from build123d import *

# Parameters (mm, degrees)
F2_R = 15
F3_R = 2


with BuildPart() as f1:
    # F0 (on Front) → F1 (revolve)
    with BuildSketch(Plane.XZ):
        Polygon((-36, -25), (-32.5, -25), (-32.5, -5), (-25.5, 5), (-25.5, 25), (-29, 25), (-29, 5), (-36, -5), align=None)
    revolve(axis=Axis((0, 0, 12.5), (0, 0, 1)))

    # F2
    f2_edges = [f1.edges().sort_by_distance(p)[0] for p in [
        (29, 0, 5),
        (36, 0, -5),
        (25.5, 0, 5),
        (32.5, 0, -5),
    ]]
    fillet(f2_edges, radius=F2_R)

    # F3
    f3_edges = [f1.edges().sort_by_distance(p)[0] for p in [
        (29, 0, 25),
    ]]
    fillet(f3_edges, radius=F3_R)


solid = f1.part
Part model, mm, in its own coordinate system. A direction names the side the tool comes from. Give positions to 0.01 mm unless a question says otherwise; leave off trailing zeros. Loops run counter-clockwise (first coordinate to the right, second up) from the corner with the lowest first, then second, coordinate; pieces in that order, holes last.
(1) Pin check, flat tips, straight feed: pin 1 (3 mm diameter, centred on x = 8, z = -9, fed in from +Y); pin 2 (10 mm diameter, centred on y = 8.5, z = 5.5, fed in from +X); pin 3 (1 mm diameter, centred on x = 7.5, z = 3.5, fed in from -Y). Stop position of each tip, or through.
Return value:
pin 1: stops at y = 35.4
pin 2: stops at x = 31.21
pin 3: stops at y = -29.69
(2) Band-saw the part on A-A (z = 19.5). Write the cut outline in (x, y).
Return value:
outline: circle Ø58 at (0, 0); hole circle Ø51 at (0, 0)
(3) Drill centre lines: line 1 along X through (y, z) = (0, 18.75); line 2 along X through (y, z) = (0, -17.25). Where is each one in solid material? Low to high.
Return value:
line 1: x = -29 to -25.5, 25.5 to 29
line 2: x = -36 to -32.5, 32.5 to 36
(4) Pull direction X, two halves, no side cores. Call faces 3 (the cylindrical face through (7.045, 31.727, -17.257)), 4 (the cylindrical face through (-34.34, -10.81, -17.47)), 5 (the flat face through (24, 10, 25)): pulls with the +X half, pulls with the -X half, needs draft (parallel to the pull), parting line crosses it, or undercut.
Return value:
face 3: undercut
face 4: parting line crosses it
face 5: needs draft
(5) 3-axis set-ups, long thin cutter, end or side, ignore diameter. For faces 1 (the cylindrical face through (5.5, 24.9, 17.5)), 2 (the cylindrical face through (-27.66, -8.71, 16.27)): which of +Z, -Z, +X, -X, +Y, -Y reach the whole face in a straight line?
Return value:
face 1: +Z, -Z
face 2: +Z
